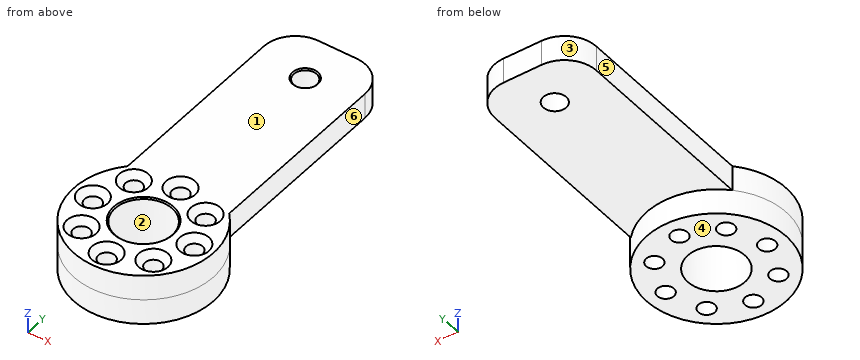
from build123d import *

# Parameters (mm, degrees)
PAD_DEPTH       = 4
SKETCH003_R     = 1.8
POCKET_DEPTH    = 5
FILLET_R        = 5
SKETCH004_R     = 11
PAD001_DEPTH    = 4
SKETCH002_R     = 4.5
SKETCH002_R_2   = 1.3
POCKET001_DEPTH = 10
CHAMFER_SIZE    = 1
CHAMFER001_SIZE = 0.2


with BuildPart() as part:
    # Sketch → Pad (new body)
    with BuildSketch(Plane.XY):
        with BuildLine():
            ThreePointArc((-8, 7.549834), (0, -11), (8, 7.549834))
            Line((8, 7.549834), (8, 42))
            Line((8, 42), (-8, 42))
            Line((-8, 42), (-8, 7.549834))
        make_face()
    extrude(amount=PAD_DEPTH)

    # Sketch003 → Pocket (cut)
    with BuildSketch(Plane.XY.offset(4)):
        with Locations((0, 35)):
            Circle(SKETCH003_R)
    extrude(amount=-POCKET_DEPTH, mode=Mode.SUBTRACT)

    # Fillet
    fillet_edges = [part.edges().sort_by_distance(p)[0] for p in [
        (-8, 42, 2),
        (8, 42, 2),
    ]]
    fillet(fillet_edges, radius=FILLET_R)

    # Sketch004 → Pad001 (join)
    with BuildSketch(Plane(origin=(0, 0, 0), x_dir=(1, 0, 0), z_dir=(0, 0, -1))):
        Circle(SKETCH004_R)
    extrude(amount=PAD001_DEPTH)

    # Sketch002 (on Face5 of Pad001) → Pocket001 (cut)
    with BuildSketch(Plane.XY.offset(4)):
        Circle(SKETCH002_R)
        with Locations((0, 8)):
            Circle(SKETCH002_R_2)
        with Locations((5.656854, 5.656854)):
            Circle(SKETCH002_R_2)
        with Locations((8, 0)):
            Circle(SKETCH002_R_2)
        with Locations((5.656854, -5.656854)):
            Circle(SKETCH002_R_2)
        with Locations((0, -8)):
            Circle(SKETCH002_R_2)
        with Locations((-5.656854, -5.656854)):
            Circle(SKETCH002_R_2)
        with Locations((-8, 0)):
            Circle(SKETCH002_R_2)
        with Locations((-5.656854, 5.656854)):
            Circle(SKETCH002_R_2)
    extrude(amount=-POCKET001_DEPTH, mode=Mode.SUBTRACT)

    # Chamfer
    chamfer_edges = [part.edges().sort_by_distance(p)[0] for p in [
        (-6.956854, 5.656854, 4),
        (-1.3, 8, 4),
        (4.356854, 5.656854, 4),
        (6.7, 0, 4),
        (4.356854, -5.656854, 4),
        (-1.3, -8, 4),
        (-6.956854, -5.656854, 4),
        (-9.3, 0, 4),
    ]]
    chamfer(chamfer_edges, length=CHAMFER_SIZE)

    # Chamfer001
    chamfer001_edges = [part.edges().sort_by_distance(p)[0] for p in [
        (-1.8, 35, 4),
        (-4.5, 0, 4),
    ]]
    chamfer(chamfer001_edges, length=CHAMFER001_SIZE)


solid = part.part
The model under review builds one solid part; all positions refer to its coordinate system, in mm. Face numbers are marked on the shaded views. A direction names the side the tool comes from. Round coordinates to 2 decimals unless told otherwise and drop trailing zeros. Loops run counter-clockwise (first coordinate to the right, second up) from the corner with the lowest first, then second, coordinate; pieces in that order, holes last. Notation, with made-up numbers: M -24.75,-6.75 L -19.75,-6.75 A17 cw -19.75,13.25 Z; hole C 34,-13 d1. An arc over 180 degrees is marked long. Answer as CSV lines item,"result".
1. We need section A-A (y = 0). Give the boundary of the cut face in (x, z), plus the area to 3 significant figures.
Outcome:
outline,"M -11,-4 L -9.3,-4 L -9.3,3 L -10.3,4 L -11,4 Z; M -6.7,-4 L -4.5,-4 L -4.5,3.8 L -4.7,4 L -5.7,4 L -6.7,3 Z; M 4.5,-4 L 6.7,-4 L 6.7,3 L 5.7,4 L 4.7,4 L 4.5,3.8 Z; M 9.3,-4 L 11,-4 L 11,4 L 10.3,4 L 9.3,3 Z"
area,"60.4 mm2"
2. We need section B-B (y = 35). Give the boundary of the cut face in (x, z), plus the area to 3 significant figures.
Outcome:
outline,"M -8,0 L -1.8,0 L -1.8,3.8 L -2,4 L -8,4 Z; M 1.8,0 L 8,0 L 8,4 L 2,4 L 1.8,3.8 Z"
area,"49.6 mm2"
3. To check wall thickness, follow L1, parallel to Y at x = 0, z = -2.5; L2, parallel to Y at x = 0, z = 1.45; L3, parallel to Y at x = 1, z = -0.5. State the ranges of each line that lie inside material, in increasing order. Write a range as [from, to].
Outcome:
L1,"y = [-11, -9.3], [-6.7, -4.5], [4.5, 6.7], [9.3, 11]"
L2,"y = [-11, -9.3], [-6.7, -4.5], [4.5, 6.7], [9.3, 33.2], [36.8, 42]"
L3,"y = [-10.95, -8.83], [-7.17, -4.39], [4.39, 7.17], [8.83, 10.95]"
4. We need section C-C (z = 0.75). Count the separate pieces of the cut face and the enclosed holes in it, plus the area to 3 significant figures.
Outcome:
separate pieces,"1"
enclosed holes,"10"
area,"766 mm2"
5. For the marked faces 4, 5 and 6, list the 3-axis set-ups (+Z, -Z, +X, -X, +Y, -Y) from which the entire face can be reached by the end or side of a thin tool; tool diameter is ignored.
Outcome:
face 4,"-Z, +X, -X, +Y, -Y"
face 5,"+Z, -Z, -X, +Y"
face 6,"+Z, -Z, +X, +Y"
6. Insertion check: pin 1 Ø2.5 at (x, y) = (-5.66, -5.66) entering from -Z; pin 2 Ø2 at (y, z) = (16.5, 2) entering from -X; pin 3 Ø5 at (x, y) = (3, 30.5) entering from -Z; pin 4 Ø2 at (y, z) = (26, 2.5) entering from +X. Each pin has a flat end and moves straight along its axis. Give the tip position at first contact, or say it passes through.
Outcome:
pin 1,"passes through"
pin 2,"stops at x = -8"
pin 3,"stops at z = 0"
pin 4,"stops at x = 8"
7. Draft analysis for pull direction Y (two halves, no side actions). For the marked faces 1, 2 and 3, state which applies: pulls with the +Y half, pulls with the -Y half, needs draft (parallel to the pull), parting line crosses it, or undercut.
Outcome:
face 1,"needs draft"
face 2,"undercut"
face 3,"pulls with the +Y half"
